Input: part model. Units: mm. Frame: model coordinates. A direction names the side the tool comes from. Coordinates: 2 decimals unless noted, no trailing zeros. Order: outer loops, then holes, each group sorted by start corner. A loop starts at its lowest first (then second) coordinate and runs counter-clockwise, first axis right, second up. Notation, with made-up numbers: M -30,42.25 L -6,42.25 A29 cw -6,79.25 Z; hole C -6.5,83.5 d10. An arc over 180 degrees is marked long. Answer in a Markdown table with one row per item.
from build123d import *

# Parameters (mm, degrees)
SKETCH1_W           = 107.95
SKETCH1_H           = 120.65
SKETCH1_R           = 3.5
SKETCH1_R_2         = 1
SKETCH1_R_3         = 1.5
SKETCH1_R_4         = 1.6999966
SKETCH1_W_2         = 48
SKETCH1_H_2         = 35
SKETCH1_W_3         = 10.5
SKETCH1_H_3         = 10.5
BOSS_EXTRUDE1_DEPTH = 2.54
FILLET1_R           = 6.35


with BuildPart() as part:
    # Sketch1 → Boss-Extrude1 (new body)
    with BuildSketch(Plane(origin=(0, 0, 0), x_dir=(1, 0, 0), z_dir=(0, 1, 0))):
        Rectangle(SKETCH1_W, SKETCH1_H)
        with Locations(Location((-38.1, 31.75, 0), (0, 0, 270))):
            Circle(SKETCH1_R, mode=Mode.SUBTRACT)
        with Locations(Location((-26.5, 46.75, 0), (0, 0, 270))):
            Circle(SKETCH1_R_2, mode=Mode.SUBTRACT)
        with Locations(Location((26.5, 46.75, 0), (0, 0, 270))):
            Circle(SKETCH1_R_2, mode=Mode.SUBTRACT)
        with Locations(Location((26.5, 16.75, 0), (0, 0, 270))):
            Circle(SKETCH1_R_2, mode=Mode.SUBTRACT)
        with Locations(Location((-26.5, 16.75, 0), (0, 0, 270))):
            Circle(SKETCH1_R_2, mode=Mode.SUBTRACT)
        with Locations(Location((-45.9, 31.75, 0), (0, 0, 270))):
            Circle(SKETCH1_R_3, mode=Mode.SUBTRACT)
        with Locations(Location((-41.275, 8.007058824, 0), (0, 0, 270))):
            Circle(SKETCH1_R_4, mode=Mode.SUBTRACT)
        with Locations(Location((41.275, 8.007058824, 0), (0, 0, 270))):
            Circle(SKETCH1_R_4, mode=Mode.SUBTRACT)
        with Locations(Location((41.275, -47.872941176, 0), (0, 0, 270))):
            Circle(SKETCH1_R_4, mode=Mode.SUBTRACT)
        with Locations(Location((-41.275, -47.872941176, 0), (0, 0, 270))):
            Circle(SKETCH1_R_4, mode=Mode.SUBTRACT)
        with Locations((0, 31.75)):
            Rectangle(SKETCH1_W_2, SKETCH1_H_2, mode=Mode.SUBTRACT)
        with Locations((30.48, -40.252941176)):
            Rectangle(SKETCH1_W_3, SKETCH1_H_3, mode=Mode.SUBTRACT)
        with Locations((-30.48, -22.472941176)):
            Rectangle(SKETCH1_W_3, SKETCH1_H_3, mode=Mode.SUBTRACT)
        with Locations((-10.16, -22.472941176)):
            Rectangle(SKETCH1_W_3, SKETCH1_H_3, mode=Mode.SUBTRACT)
        with Locations((10.16, -22.472941176)):
            Rectangle(SKETCH1_W_3, SKETCH1_H_3, mode=Mode.SUBTRACT)
        with Locations((30.48, -22.472941176)):
            Rectangle(SKETCH1_W_3, SKETCH1_H_3, mode=Mode.SUBTRACT)
        with Locations((10.16, -40.252941176)):
            Rectangle(SKETCH1_W_3, SKETCH1_H_3, mode=Mode.SUBTRACT)
        with Locations((-10.16, -40.252941176)):
            Rectangle(SKETCH1_W_3, SKETCH1_H_3, mode=Mode.SUBTRACT)
        with Locations((-30.48, -40.252941176)):
            Rectangle(SKETCH1_W_3, SKETCH1_H_3, mode=Mode.SUBTRACT)
        Rectangle(SKETCH1_W_3, SKETCH1_H_3, mode=Mode.SUBTRACT)
        with Locations((-15.41, 0)):
            Rectangle(SKETCH1_W_3, SKETCH1_H_3, mode=Mode.SUBTRACT)
        with Locations((15.41, 0)):
            Rectangle(SKETCH1_W_3, SKETCH1_H_3, mode=Mode.SUBTRACT)
    extrude(amount=BOSS_EXTRUDE1_DEPTH)

    # Fillet1
    fillet1_edges = [part.edges().sort_by_distance(p)[0] for p in [
        (53.975, 1.27, 60.325),
        (-53.975, 1.27, 60.325),
        (-53.975, 1.27, -60.325),
        (53.975, 1.27, -60.325),
    ]]
    fillet(fillet1_edges, radius=FILLET1_R)


solid = part.part
1) Contact query for a flat-ended pin moving along its axis: pin 1 (1.2 mm diameter, centred on x = 26.5, z = -16.75, fed in from -Y). Output: stop coordinate, or through.
Resolved:
| item | result |
|---|---|
| pin 1 | passes through |
2) Mould query, pull axis X, two halves, no side actions, for faces 3 (the face through (-52.16, 1.29, 58.42)), 4 (the face through (10, 1, 45.503)), 5 (the face through (20.66, 1, 0)), 6 (the face through (52.07, 1.29, 58.51)). Classes: +X half, -X half, draft (parallel to the pull), parting line (faces both ways), or undercut.
Resolved:
| item | result |
|---|---|
| face 3 | -X half |
| face 4 | undercut |
| face 5 | undercut |
| face 6 | +X half |
3) Reachability of faces 1 (the face through (4.91, 1, 40)), 2 (the face through (-52.16, 1.29, -58.42)) from +Z, -Z, +X, -X, +Y, -Y: full face, straight path, thin tool, end or side. Return the list, or none.
Resolved:
| item | result |
|---|---|
| face 1 | +Y, -Y |
| face 2 | -Z, -X, +Y, -Y |
4) Cut plane B-B, the plane z = -43. Output: boundary loops of the cut face in (x, y) (3 decimals), and give its area (3 significant figures).
Resolved:
| item | result |
|---|---|
| outline | M -53.975,0 L -24,0 L -24,2.54 L -53.975,2.54 Z; M 24,0 L 53.975,0 L 53.975,2.54 L 24,2.54 Z |
| area | 152 mm2 |
5) Cut plane C-C, the plane x = -38.1. Output: boundary loops of the cut face in (y, z) (3 decimals).
Resolved:
| item | result |
|---|---|
| outline | M 0,-60.325 L 2.54,-60.325 L 2.54,-35.25 L 0,-35.25 Z; M 0,-28.25 L 2.54,-28.25 L 2.54,60.325 L 0,60.325 Z |
6) Cut plane D-D, the plane z = -2.5. Output: boundary loops of the cut face in (x, y) (3 decimals), and give its area (3 significant figures).
Resolved:
| item | result |
|---|---|
| outline | M -53.975,0 L -20.66,0 L -20.66,2.54 L -53.975,2.54 Z; M -10.16,0 L -5.25,0 L -5.25,2.54 L -10.16,2.54 Z; M 5.25,0 L 10.16,0 L 10.16,2.54 L 5.25,2.54 Z; M 20.66,0 L 53.975,0 L 53.975,2.54 L 20.66,2.54 Z |
| area | 194 mm2 |
7) Cut plane A-A, the plane x = 12.5. Output: boundary loops of the cut face in (y, z) (3 decimals), and give its area (3 significant figures).
Resolved:
| item | result |
|---|---|
| outline | M 0,-60.325 L 2.54,-60.325 L 2.54,-49.25 L 0,-49.25 Z; M 0,-14.25 L 2.54,-14.25 L 2.54,-5.25 L 0,-5.25 Z; M 0,5.25 L 2.54,5.25 L 2.54,17.223 L 0,17.223 Z; M 0,27.723 L 2.54,27.723 L 2.54,35.003 L 0,35.003 Z; M 0,45.503 L 2.54,45.503 L 2.54,60.325 L 0,60.325 Z |
| area | 138 mm2 |
8) Material intervals for probe 1 along Z at (x, y) = (20, 1.9) (3 decimals); probe 2 along Z at (x, y) = (-5, 1.75) (3 decimals); probe 3 along X at (y, z) = (0.95, -46.75) (3 decimals), sorted ascending.
Resolved:
| item | result |
|---|---|
| probe 1 | z = -60.325 to -49.25, -14.25 to -5.25, 5.25 to 60.325 |
| probe 2 | z = -60.325 to -49.25, -14.25 to -5.25, 5.25 to 17.223, 27.723 to 35.003, 45.503 to 60.325 |
| probe 3 | x = -53.975 to -27.5, -25.5 to -24, 24 to 25.5, 27.5 to 53.975 |
